from build123d import *

# Parameters (mm, degrees)
SKETCH_1_W                     = 50
SKETCH_1_H                     = 100
EXTRUDE_1_DEPTH                = 2
SKETCH_2_W                     = 3
SKETCH_2_H                     = 100
EXTRUDE_2_DEPTH                = 80
SKETCH_3_W                     = 2
SKETCH_3_H                     = 66.7
EXTRUDE_3_DEPTH                = 70
CUT_EXTRUDE_4_REACH            = 162.465
SKETCH_8_W                     = 2
SKETCH_8_H                     = 66.7
EXTRUDE_4_DEPTH                = 70
CUT_EXTRUDE_5_REACH            = 140.25
HOLE_WIZARD_M3_1_D             = 2.5
HOLE_WIZARD_M3_1_DEPTH         = 2
HOLE_WIZARD_M3_1_CSINK_D       = 3.05
HOLE_WIZARD_M3_1_CSINK_ANGLE   = 90
FILLET_1_R                     = 2
CUT_EXTRUDE_6_REACH            = 140.25
SKETCH_12_R                    = 11
CUT_EXTRUDE_7_REACH            = 162.465
SKETCH_13_R                    = 14.5
SKETCH_14_W                    = 2
SKETCH_14_H                    = 66.7
EXTRUDE_5_DEPTH                = 70
CUT_EXTRUDE_8_REACH            = 156.14
SKETCH_15_R                    = 5.1
CUT_EXTRUDE_9_DEPTH            = 155.140358116
CUT_EXTRUDE_9_DEPTH_BACK       = 155.140358116
SKETCH_19_W                    = 2
SKETCH_19_H                    = 66.7
CUT_EXTRUDE_10_DEPTH           = 119.844436134
FILLET_2_R                     = 2
CUT_EXTRUDE_12_DEPTH           = 134.88427839
CUT_EXTRUDE_12_DEPTH_BACK      = 134.88427839
SKETCH_20_W                    = 47
SKETCH_20_H                    = 100
SKETCH_20_W_2                  = 70
SKETCH_20_H_2                  = 2
HOLE_WIZARD_M2_5_1_D           = 2.05
HOLE_WIZARD_M2_5_1_CSINK_D     = 2.55
HOLE_WIZARD_M2_5_1_CSINK_ANGLE = 90
SKETCH_23_W                    = 70
SKETCH_23_H                    = 10
CUT_EXTRUDE_13_DEPTH           = 97.088500873
FILLET_3_R                     = 0.8
FILLET_4_R                     = 0.8


with BuildPart() as part:
    # 草图1 → 凸台-拉伸1 (new body)
    with BuildSketch(Plane(origin=(0, 0, 0), x_dir=(1, 0, 0), z_dir=(0, 1, 0))):
        Rectangle(SKETCH_1_W, SKETCH_1_H)
    extrude(amount=EXTRUDE_1_DEPTH)

    # 草图2 → 凸台-拉伸2 (add)
    with BuildSketch(Plane(origin=(0, 2, 0), x_dir=(1, 0, 0), z_dir=(0, 1, 0))):
        with Locations((-23.5, 0)):
            Rectangle(SKETCH_2_W, SKETCH_2_H)
    extrude(amount=EXTRUDE_2_DEPTH)

    # 草图3 → 凸台-拉伸3 (add)
    with BuildSketch(Plane.ZY.offset(25)):
        with Locations((-49, 48.65)):
            Rectangle(SKETCH_3_W, SKETCH_3_H)
    extrude(amount=EXTRUDE_3_DEPTH)

    # 草图4 → 切除-拉伸4 (cut, up to next)
    with BuildSketch(Plane(origin=(0, 0, -50), x_dir=(-1, 0, 0), z_dir=(0, 0, -1)), mode=Mode.PRIVATE) as cut_extrude_4_sk1:
        with BuildLine():
            Line((95, 82), (61.65, 82))
            ThreePointArc((61.65, 82), (85.232011153, 72.232011153), (95, 48.65))
            Line((95, 48.65), (95, 82))
        make_face()
    cut_extrude_4_tool1 = extrude(cut_extrude_4_sk1.sketch, amount=-CUT_EXTRUDE_4_REACH, mode=Mode.PRIVATE) & part.part
    # 草图4 → 切除-拉伸4 (cut, up to next)
    with BuildSketch(Plane(origin=(0, 0, -50), x_dir=(-1, 0, 0), z_dir=(0, 0, -1)), mode=Mode.PRIVATE) as cut_extrude_4_sk2:
        with BuildLine():
            ThreePointArc((95, 48.65), (85.232011153, 25.067988847), (61.65, 15.3))
            Line((61.65, 15.3), (95, 15.3))
            Line((95, 15.3), (95, 48.65))
        make_face()
    cut_extrude_4_tool2 = extrude(cut_extrude_4_sk2.sketch, amount=-CUT_EXTRUDE_4_REACH, mode=Mode.PRIVATE) & part.part
    add(cut_extrude_4_tool1.solids().sort_by_distance((-87.550679, 74.550679, -50))[0], mode=Mode.SUBTRACT)
    add(cut_extrude_4_tool2.solids().sort_by_distance((-87.550679, 22.749321, -50))[0], mode=Mode.SUBTRACT)

    # 草图8 → 凸台-拉伸4 (add)
    with BuildSketch(Plane.ZY.offset(25)):
        with Locations((7, 48.65)):
            Rectangle(SKETCH_8_W, SKETCH_8_H)
    extrude(amount=EXTRUDE_4_DEPTH)

    # 草图9 → 切除-拉伸5 (cut, up to next)
    with BuildSketch(Plane.XY.offset(8), mode=Mode.PRIVATE) as cut_extrude_5_sk1:
        with BuildLine():
            ThreePointArc((-95, 48.65), (-85.232011153, 72.232011153), (-61.65, 82))
            Line((-61.65, 82), (-95, 82))
            Line((-95, 82), (-95, 48.65))
        make_face()
    cut_extrude_5_tool1 = extrude(cut_extrude_5_sk1.sketch, amount=-CUT_EXTRUDE_5_REACH, mode=Mode.PRIVATE) & part.part
    # 草图9 → 切除-拉伸5 (cut, up to next)
    with BuildSketch(Plane.XY.offset(8), mode=Mode.PRIVATE) as cut_extrude_5_sk2:
        with BuildLine():
            ThreePointArc((-61.65, 15.3), (-85.232011153, 25.067988847), (-95, 48.65))
            Line((-95, 48.65), (-95, 15.3))
            Line((-95, 15.3), (-61.65, 15.3))
        make_face()
    cut_extrude_5_tool2 = extrude(cut_extrude_5_sk2.sketch, amount=-CUT_EXTRUDE_5_REACH, mode=Mode.PRIVATE) & part.part
    add(cut_extrude_5_tool1.solids().sort_by_distance((-87.550679, 74.550679, 8))[0], mode=Mode.SUBTRACT)
    add(cut_extrude_5_tool2.solids().sort_by_distance((-87.550679, 22.749321, 8))[0], mode=Mode.SUBTRACT)

    # M3 螺纹孔1
    with Locations(Plane.XY.offset(8)):
        with Locations((-78.970508076, 38.65), (-61.65, 68.65), (-44.329491924, 38.65)):
            CounterSinkHole(HOLE_WIZARD_M3_1_D / 2, HOLE_WIZARD_M3_1_CSINK_D / 2, depth=HOLE_WIZARD_M3_1_DEPTH, counter_sink_angle=HOLE_WIZARD_M3_1_CSINK_ANGLE)

    # 圆角1
    fillet_1_edges = [part.edges().sort_by_distance(p)[0] for p in [
        (-23.5, 82, 50),
        (25, 1, 50),
        (25, 1, -50),
    ]]
    fillet(fillet_1_edges, radius=FILLET_1_R)

    # 草图12 → 切除-拉伸6 (cut, up to next)
    with BuildSketch(Plane.XY.offset(8), mode=Mode.PRIVATE) as cut_extrude_6_sk1:
        with Locations((-61.65, 48.65)):
            Circle(SKETCH_12_R)
    cut_extrude_6_tool1 = extrude(cut_extrude_6_sk1.sketch, amount=-CUT_EXTRUDE_6_REACH, mode=Mode.PRIVATE) & part.part
    add(cut_extrude_6_tool1.solids().sort_by_distance((-61.65, 48.65, 8))[0], mode=Mode.SUBTRACT)

    # 草图13 → 切除-拉伸7 (cut, up to next)
    with BuildSketch(Plane(origin=(0, 0, -50), x_dir=(-1, 0, 0), z_dir=(0, 0, -1)), mode=Mode.PRIVATE) as cut_extrude_7_sk1:
        with Locations((61.65, 48.65)):
            Circle(SKETCH_13_R)
    cut_extrude_7_tool1 = extrude(cut_extrude_7_sk1.sketch, amount=-CUT_EXTRUDE_7_REACH, mode=Mode.PRIVATE) & part.part
    add(cut_extrude_7_tool1.solids().sort_by_distance((-61.65, 48.65, -50))[0], mode=Mode.SUBTRACT)

    # 草图14 → 凸台-拉伸5 (add)
    with BuildSketch(Plane.ZY.offset(25)):
        with Locations((-38.5, 48.65)):
            Rectangle(SKETCH_14_W, SKETCH_14_H)
    extrude(amount=EXTRUDE_5_DEPTH)

    # 草图15 → 切除-拉伸8 (cut, up to next)
    with BuildSketch(Plane(origin=(0, 0, -39.5), x_dir=(-1, 0, 0), z_dir=(0, 0, -1)), mode=Mode.PRIVATE) as cut_extrude_8_sk1:
        with Locations(Location((61.65, 48.65, 0), (0, 0, 90))):
            Circle(SKETCH_15_R)
    cut_extrude_8_tool1 = extrude(cut_extrude_8_sk1.sketch, amount=-CUT_EXTRUDE_8_REACH, mode=Mode.PRIVATE) & part.part
    add(cut_extrude_8_tool1.solids().sort_by_distance((-61.65, 48.65, -39.5))[0], mode=Mode.SUBTRACT)

    # 草图18 → 切除-拉伸9 (cut, two sides: drawn at the far end of the back side and taken through both)
    with BuildSketch(Plane(origin=(0, 0, -39.5), x_dir=(-1, 0, 0), z_dir=(0, 0, -1)).offset(-CUT_EXTRUDE_9_DEPTH_BACK)):
        with BuildLine():
            Line((95, 15.3), (95, 48.65))
            ThreePointArc((95, 48.65), (85.232011153, 25.067988847), (61.65, 15.3))
            Line((61.65, 15.3), (95, 15.3))
        make_face()
        with BuildLine():
            Line((95, 48.65), (95, 82))
            Line((95, 82), (61.65, 82))
            ThreePointArc((61.65, 82), (85.232011153, 72.232011153), (95, 48.65))
        make_face()
    extrude(amount=CUT_EXTRUDE_9_DEPTH + CUT_EXTRUDE_9_DEPTH_BACK, mode=Mode.SUBTRACT)

    # 草图19 → 切除-拉伸10 (cut, through all)
    with BuildSketch(Plane.ZY.offset(25)):
        with Locations((-49, 48.65)):
            Rectangle(SKETCH_19_W, SKETCH_19_H)
    extrude(amount=CUT_EXTRUDE_10_DEPTH, mode=Mode.SUBTRACT)

    # 圆角2
    fillet_2_edges = [part.edges().sort_by_distance(p)[0] for p in [
        (-23.5, 82, -50),
    ]]
    fillet(fillet_2_edges, radius=FILLET_2_R)

    # 草图20 → 切除-拉伸12 (cut, two sides: drawn at the far end of the back side and taken through both)
    with BuildSketch(Plane(origin=(0, 2, 0), x_dir=(1, 0, 0), z_dir=(0, 1, 0)).offset(-CUT_EXTRUDE_12_DEPTH_BACK)):
        with Locations((1.5, 0)):
            Rectangle(SKETCH_20_W, SKETCH_20_H)
        with Locations((-60, 38.5)):
            Rectangle(SKETCH_20_W_2, SKETCH_20_H_2)
        with Locations((-60, -7)):
            Rectangle(SKETCH_20_W_2, SKETCH_20_H_2)
    extrude(amount=CUT_EXTRUDE_12_DEPTH + CUT_EXTRUDE_12_DEPTH_BACK, mode=Mode.SUBTRACT)

    # M2.5 螺纹孔1 (through all)
    with Locations(Plane(origin=(-22, 0, 0), x_dir=(0, 0, -1), z_dir=(1, 0, 0))):
        with Locations((-2, 14), (-9, 6), (9, 6), (33.5, 57.65), (33.5, 39.65), (-2, 32)):
            CounterSinkHole(HOLE_WIZARD_M2_5_1_D / 2, HOLE_WIZARD_M2_5_1_CSINK_D / 2, counter_sink_angle=HOLE_WIZARD_M2_5_1_CSINK_ANGLE)

    # 草图23 → 切除-拉伸13 (cut, through all)
    with BuildSketch(Plane(origin=(-22, 0, 0), x_dir=(0, 0, -1), z_dir=(1, 0, 0))):
        with Locations((0, 23)):
            Rectangle(SKETCH_23_W, SKETCH_23_H)
    extrude(amount=-CUT_EXTRUDE_13_DEPTH, mode=Mode.SUBTRACT)

    # 圆角3
    fillet_3_edges = [part.edges().sort_by_distance(p)[0] for p in [
        (-22, 82, 0),
        (-22, 40, 50),
        (-22, 81.414213562, 49.414213562),
        (-25, 40, 50),
        (-25, 81.414213562, 49.414213562),
        (-25, 40, -50),
        (-25, 81.414213562, -49.414213562),
        (-22, 40, -50),
        (-22, 81.414213562, -49.414213562),
        (-25, 23, 35),
        (-25, 28, 0),
        (-23.5, 28, 35),
        (-25, 23, -35),
        (-23.5, 28, -35),
        (-25, 18, 0),
        (-22, 23, 35),
        (-22, 18, 0),
        (-22, 23, -35),
        (-22, 28, 0),
        (-25, 82, 0),
    ]]
    fillet(fillet_3_edges, radius=FILLET_3_R)

    # 圆角4
    fillet_4_edges = [part.edges().sort_by_distance(p)[0] for p in [
        (-25, 0, 0),
        (-22, 0, 0),
        (-23.5, 0, 50),
        (-23.5, 0, -50),
        (-22.234314575, 0, -49.765685425),
        (-24.765685425, 0, -49.765685425),
        (-22.234314575, 0, 49.765685425),
        (-24.765685425, 0, 49.765685425),
    ]]
    fillet(fillet_4_edges, radius=FILLET_4_R)


solid = part.part
Check sheet for the modelled part. Datum: model origin and axes. Units: mm. Round coordinates to 2 decimals unless told otherwise and drop trailing zeros. Write each loop counter-clockwise with the first axis right and the second up, starting at its lowest first coordinate (ties: lowest second). Pieces come first, ordered by that corner, then holes. Notation, with made-up numbers: (22, 18) - (45, 18) arc R11 cw to (45, 35) - close; hole circle Ø2 at (70.5, 47). An arc over 180 degrees is marked (long way). Return JSON: item names as keys, results as strings.
Q1. Draft check along Y on faces 1 (the cylindrical face through (-23.49, 81.43, 49.4)), 2 (the flat face through (-25, 42, -1)), 3 (the cylindrical face through (-23.644, 33.016, 1.867)). Enter one of: released by +Y, released by -Y, zero draft, split by the parting line, or undercut.
Returned:
{"face 1": "released by +Y", "face 2": "zero draft", "face 3": "undercut"}
Q2. Cross-section at A-A (x = -23.5). Record the boundary of the cut face in (y, z) (3 decimals).
Returned:
{"outline": "(0, -49.2) arc R0.8 ccw to (0.8, -50) - (80, -50) arc R2 ccw to (82, -48) - (82, 48) arc R2 ccw to (80, 50) - (0.8, 50) arc R0.8 ccw to (0, 49.2) - close; hole circle Ø2.05 at (6, -9); hole circle Ø2.05 at (6, 9); hole circle Ø2.05 at (14, 2); hole (18, -35) - (27.2, -35) arc R0.8 ccw to (28, -34.2) - (28, 34.2) arc R0.8 ccw to (27.2, 35) - (18, 35) - close; hole circle Ø2.05 at (32, 2); hole circle Ø2.05 at (39.65, -33.5); hole circle Ø2.05 at (57.65, -33.5)"}
Q3. Depth check by flat-ended pin: P1, Ø2.5, axis at y = 32, z = 2, coming from the -X side; P2, Ø2.5, axis at y = 39.65, z = -33.5, coming from the +X side (3 decimals); P3, Ø1.8, axis at y = 6, z = 9, coming from the -X side. Enter the tip coordinate at first touch or a pass-through.
Returned:
{"P1": "stops at x = -25", "P2": "stops at x = -22.025", "P3": "passes through"}
Q4. Scan lines: L1, parallel to Y at x = -24.2, z = -9 (3 decimals); L2, parallel to Y at x = -24.2, z = -33.5 (3 decimals); L3, parallel to Y at x = -22.8, z = -16. Record each from-to range of solid material in increasing order. Write a range as from..to.
Returned:
{"L1": "y = 0..4.975, 7.025..18, 28..82", "L2": "y = 0..18, 28..38.625, 40.675..56.625, 58.675..82", "L3": "y = 0..18, 28..82"}
Q5. Cross-section at B-B (z = -13). Record the boundary of the cut face in (x, y).
Returned:
{"outline": "(-25, 0.8) arc R0.8 ccw to (-24.2, 0) - (-22.8, 0) arc R0.8 ccw to (-22, 0.8) - (-22, 17.2) arc R0.8 ccw to (-22.8, 18) - (-24.2, 18) arc R0.8 ccw to (-25, 17.2) - close; (-25, 28.8) arc R0.8 ccw to (-24.2, 28) - (-22.8, 28) arc R0.8 ccw to (-22, 28.8) - (-22, 81.2) arc R0.8 ccw to (-22.8, 82) - (-24.2, 82) arc R0.8 ccw to (-25, 81.2) - close"}
